The listing builds one solid part. Answer for the finished solid, in the listing's coordinates (mm). A direction names the side the tool comes from. Round coordinates to 2 decimals unless told otherwise and drop trailing zeros. Write each loop counter-clockwise with the first axis right and the second up, starting at its lowest first coordinate (ties: lowest second). Pieces come first, ordered by that corner, then holes. Notation, with made-up numbers: (-24, 65.25) -> (4, 65.25) arc R26 cw to (4, 91.25) -> close; hole circle Ø6 at (38, -6.75). An arc over 180 degrees is marked (long way). Write each question's results on one line, items separated by ' | '. Start each with the question number.
```python
from build123d import *

# Parameters (mm, degrees)
SKETCH3_W           = 30
SKETCH3_H           = 30
BOSS_EXTRUDE1_DEPTH = 30
SKETCH4_R           = 15
SKETCH4_R_2         = 6
BOSS_EXTRUDE2_DEPTH = 40
SKETCH5_R           = 15
BOSS_EXTRUDE3_DEPTH = 40
CUT_EXTRUDE4_DEPTH  = 40
SKETCH7_R           = 3
BOSS_EXTRUDE4_DEPTH = 1
SKETCH8_R           = 4.5
BOSS_EXTRUDE5_DEPTH = 1
CUT_EXTRUDE5_DEPTH  = 0.5
SKETCH10_R          = 6
BOSS_EXTRUDE6_DEPTH = 428
FILLET1_R           = 1


with BuildPart() as part:
    # Sketch3 → Boss-Extrude1 (new body)
    with BuildSketch(Plane.XY):
        with Locations((15, 15)):
            Rectangle(SKETCH3_W, SKETCH3_H)
    extrude(amount=BOSS_EXTRUDE1_DEPTH)

    # Sketch4 → Boss-Extrude2 (add)
    with BuildSketch(Plane.XY.offset(30)):
        with Locations((15, 15)):
            Circle(SKETCH4_R)
        with Locations((15, 15)):
            Circle(SKETCH4_R_2, mode=Mode.SUBTRACT)
    extrude(amount=BOSS_EXTRUDE2_DEPTH)

    # Sketch5 → Boss-Extrude3 (add)
    with BuildSketch(Plane.XZ):
        with Locations((15, 15)):
            Circle(SKETCH5_R)
    extrude(amount=BOSS_EXTRUDE3_DEPTH)

    # Sketch6 → Cut-Extrude4 (cut)
    with BuildSketch(Plane.XZ.offset(40)):
        with BuildLine():
            Line((6, 27), (24, 27))
            ThreePointArc((24, 27), (15, 30), (6, 27))
        make_face()
    extrude(amount=-CUT_EXTRUDE4_DEPTH, mode=Mode.SUBTRACT)

    # Sketch7 → Boss-Extrude4 (add)
    with BuildSketch(Plane.XY.offset(27)):
        with Locations((15, -21.5)):
            Circle(SKETCH7_R)
    extrude(amount=BOSS_EXTRUDE4_DEPTH)

    # Sketch8 → Boss-Extrude5 (add)
    with BuildSketch(Plane.XY.offset(28)):
        with Locations((15, -21.5)):
            Circle(SKETCH8_R)
    extrude(amount=BOSS_EXTRUDE5_DEPTH)

    # Sketch9 → Cut-Extrude5 (cut)
    with BuildSketch(Plane.XY.offset(29)):
        with BuildLine():
            Line((16.2, -17.162950312), (16.2, -25.837049688))
            ThreePointArc((16.2, -25.837049688), (15, -26), (13.8, -25.837049688))
            Line((13.8, -25.837049688), (13.8, -17.162950312))
            ThreePointArc((13.8, -17.162950312), (15, -17), (16.2, -17.162950312))
        make_face()
    extrude(amount=-CUT_EXTRUDE5_DEPTH, mode=Mode.SUBTRACT)

    # Sketch10 → Boss-Extrude6 (add)
    with BuildSketch(Plane.XZ.offset(40)):
        with Locations((15, 15)):
            Circle(SKETCH10_R)
    extrude(amount=BOSS_EXTRUDE6_DEPTH)

    # Fillet1
    fillet1_edges = [part.edges().sort_by_distance(p)[0] for p in [
        (9, -468, 15),
    ]]
    fillet(fillet1_edges, radius=FILLET1_R)


solid = part.part
```
Q1. Each of these flat-tipped pins is pushed along its axis until it touches: pin 1 (4 mm diameter, centred on x = 4.5, z = 52, fed in from -Y); pin 2 (1 mm diameter, centred on x = 17.5, y = -130.5, fed in from -Z); pin 3 (6 mm diameter, centred on y = -59, z = 17.5, fed in from +X). Where does it stop, or does it pass through?
Q2. The part is cut by section B-B, the plane y = -32. Write down the section's boundary in (x, z), then the cut area to 3 significant figures.
Q3. Find the intervals of material crossed by line 1 (Y direction, x = 15, z = 52); line 2 (Z direction, x = 16, y = -420); line 3 (Z direction, x = 19, y = -275.5), in increasing order.
Q4. Determine the mould class of faces 1 (the flat face through (19, -20, 27)), 2 (the cylindrical face through (20.54, -250.51, 12.7)), 3 (the flat face through (26, 0, 3)) for opening direction Y: pulls with the +Y half, pulls with the -Y half, needs draft (parallel to the pull), parting line crosses it, or undercut.
Q5. The part is cut by section A-A, the plane y = -434.5. Write down the section's boundary in (x, z), then the cut area to 3 significant figures.
Q6. For faces 4 (the cylindrical face through (20.54, 12.7, 49.72)), 5 (the flat face through (3, 0, 4)), 6 (the flat face through (3, 4, 30)), determine the directions among +Z, -Z, +X, -X, +Y, -Y from which every point of the face is accessible in a straight line to the end or side of a thin tool.
Answers follow:
1) pin 1: y = 2.64 | pin 2: z = 9.34 | pin 3: x = 21
2) outline: (6, 27) arc R15 ccw (long way) to (24, 27) -> close | area: 670 mm^2
3) line 1: 0 to 9, 21 to 30 | line 2: 9.08 to 20.92 | line 3: 10.53 to 19.47
4) face 1: undercut | face 2: needs draft | face 3: pulls with the -Y half
5) outline: circle Ø12 at (15, 15) | area: 113 mm^2
6) face 4: +Z | face 5: -Z, -X, -Y | face 6: +Z, -X, -Y
